Here's how the part is built. I have some questions about the finished solid (model axes, mm). A direction names the side the tool comes from. Coordinates: 2 decimals unless noted, no trailing zeros. Write each loop counter-clockwise with the first axis right and the second up, starting at its lowest first coordinate (ties: lowest second). Pieces come first, ordered by that corner, then holes.
Item 1: If we mould it in two halves opening along Y, with no side actions, what happens to faces 4 (the face through (8, 20, 4)), 5 (the face through (-6, 37, -122)), 6 (the face through (1.52, 64.59, -103.96))? For each: pulls with the +Y half, pulls with the -Y half, needs draft (parallel to the pull), parting line crosses it, or undercut.
Item 2: I want a section at C-C (x = 11.5). Please give me the cut outline in (y, z), and give its area (3 significant figures).
Item 3: I want a section at B-B (z = -86). Please give me the cut outline in (x, y).
Item 4: Please list where these lines run through material, in increasing order: line 1 (Y direction, x = 1.75, z = -94.5); line 2 (Z direction, x = 2.5, y = 69.5); line 3 (Y direction, x = 1.4, z = -27).
Item 5: For faces 1 (the face through (1.52, 22.15, -34.3)), 2 (the face through (8, 14, 0.975)), 3 (the face through (-3, 36.7, -125.4)), which set-ups out of +Z, -Z, +X, -X, +Y, -Y let a thin tool reach every point of the face, with its end or its side?
Item 6: I want a section at A-A (y = -10.68). Please give me the cut outline in (x, z).
Item 7: I'm going to push flat-ended pins straight in: P1, Ø6.5, axis at y = 0, z = -120, coming from the +X side; P2, Ø1.8, axis at x = 9.5, z = 4.5, coming from the -Y side; P3, Ø2.5, axis at x = -2, z = -123, coming from the +Y side. Where does each tip first touch, or does it pass through?
from build123d import *

# Parameters (mm, degrees)
SKETCH_1_R          = 2
EXTRUDE_1_DEPTH     = 3
EXTRUDE_2_DEPTH     = 10
CUT_EXTRUDE_3_DEPTH = 4
CHAMFER_1_SIZE      = 1
EXTRUDE_3_DEPTH     = 6
SKETCH_11_W         = 3
SKETCH_11_H         = 14
CUT_EXTRUDE_4_DEPTH = 162.773826789
SKETCH_12_R         = 1.45
CUT_EXTRUDE_5_DEPTH = 157.648043168


with BuildPart() as part:
    # Sketch 1 → Extrude 1 (new body)
    with BuildSketch(Plane(origin=(0, 0, 0), x_dir=(0, 0, -1), z_dir=(1, 0, 0))):
        Polygon((0, -15.68), (127.277441161, -15.68), (127.277441161, 89.32), (-6.974965275, 89.32), (-6.974965275, -15.68), align=None)
        with Locations((0, -10.68)):
            Circle(SKETCH_1_R, mode=Mode.SUBTRACT)
        with Locations((27, -10.68)):
            Circle(SKETCH_1_R, mode=Mode.SUBTRACT)
        with Locations((27, 0)):
            Circle(SKETCH_1_R, mode=Mode.SUBTRACT)
        Circle(SKETCH_1_R, mode=Mode.SUBTRACT)
        with Locations((93, 0)):
            Circle(SKETCH_1_R, mode=Mode.SUBTRACT)
        with Locations((93, -10.68)):
            Circle(SKETCH_1_R, mode=Mode.SUBTRACT)
        with Locations((120, -10.68)):
            Circle(SKETCH_1_R, mode=Mode.SUBTRACT)
        with Locations((120, 0)):
            Circle(SKETCH_1_R, mode=Mode.SUBTRACT)
        with Locations((73.5, 73)):
            Circle(SKETCH_1_R, mode=Mode.SUBTRACT)
        with Locations((73.5, 83.68)):
            Circle(SKETCH_1_R, mode=Mode.SUBTRACT)
        with Locations((46.5, 83.68)):
            Circle(SKETCH_1_R, mode=Mode.SUBTRACT)
        with Locations((46.5, 73)):
            Circle(SKETCH_1_R, mode=Mode.SUBTRACT)
    extrude(amount=EXTRUDE_1_DEPTH)

    # Sketch 2 → Extrude 2 (add)
    with BuildSketch(Plane(origin=(3, 0, 0), x_dir=(0, 0, -1), z_dir=(1, 0, 0))):
        Polygon((-6.974965275, 20), (-6.974965275, 9.003796157), (-4.947379944, 9.003796157), (-0.974965275, 9.003796157), (-0.974965275, 20), (-4.947379944, 20), align=None)
    extrude(amount=EXTRUDE_2_DEPTH)

    # Sketch 9 → Cut-Extrude 3 (cut)
    with BuildSketch(Plane(origin=(3, 0, 0), x_dir=(0, 0, -1), z_dir=(1, 0, 0))):
        with BuildLine():
            Line((14.793826902, 53.360356634), (27.387336033, 65.953865765))
            ThreePointArc((27.387336033, 65.953865765), (27.387336033, 70.795026635), (22.546175163, 70.795026635))
            Line((22.546175163, 70.795026635), (9.952666032, 58.201517504))
            ThreePointArc((9.952666032, 58.201517504), (9.952666032, 53.360356634), (14.793826902, 53.360356634))
        make_face()
        with BuildLine():
            Line((20.897912876, 31.977379799), (40.129928133, 51.209395056))
            ThreePointArc((40.129928133, 51.209395056), (40.129928133, 58.660989456), (32.678333733, 58.660989456))
            Line((32.678333733, 58.660989456), (13.446318476, 39.428974199))
            ThreePointArc((13.446318476, 39.428974199), (13.446318476, 31.977379799), (20.897912876, 31.977379799))
        make_face()
        with BuildLine():
            Line((20.319435032, 8.171706676), (48.67938199, 36.531653634))
            ThreePointArc((48.67938199, 36.531653634), (48.67938199, 41.992648329), (43.218387294, 41.992648329))
            Line((43.218387294, 41.992648329), (14.858440337, 13.632701372))
            ThreePointArc((14.858440337, 13.632701372), (14.858440337, 8.171706676), (20.319435032, 8.171706676))
        make_face()
        Polygon((-6.974965275, 69.32), (13.025034725, 89.32), (-6.974965275, 89.32), align=None)
        with BuildLine():
            ThreePointArc((60.151237943, 62.780937069), (56.651237943, 59.280937069), (60.151237943, 55.780937069))
            Line((60.151237943, 55.780937069), (60.151237943, 62.780937069))
        make_face()
        with BuildLine():
            Line((60.151237943, 62.780937069), (60.151237943, 55.780937069))
            ThreePointArc((60.151237943, 55.780937069), (62.626111677, 56.806063335), (63.651237943, 59.280937069))
            ThreePointArc((63.651237943, 59.280937069), (62.626111677, 61.755810803), (60.151237943, 62.780937069))
        make_face()
        with BuildLine():
            ThreePointArc((60.151237943, 40.32), (56.651237943, 36.82), (60.151237943, 33.32))
            Line((60.151237943, 33.32), (60.151237943, 40.32))
        make_face()
        with BuildLine():
            Line((60.151237943, 40.32), (60.151237943, 33.32))
            ThreePointArc((60.151237943, 33.32), (62.626111677, 34.345126266), (63.651237943, 36.82))
            ThreePointArc((63.651237943, 36.82), (62.626111677, 39.294873734), (60.151237943, 40.32))
        make_face()
        with BuildLine():
            ThreePointArc((60.151237943, 10.666059051), (56.651237943, 7.166059051), (60.151237943, 3.666059051))
            Line((60.151237943, 3.666059051), (60.151237943, 10.666059051))
        make_face()
        with BuildLine():
            Line((60.151237943, 10.666059051), (60.151237943, 3.666059051))
            ThreePointArc((60.151237943, 3.666059051), (62.626111677, 4.691185317), (63.651237943, 7.166059051))
            ThreePointArc((63.651237943, 7.166059051), (62.626111677, 9.640932785), (60.151237943, 10.666059051))
        make_face()
        with BuildLine():
            ThreePointArc((71.623093896, 36.531653634), (71.623093896, 41.992648329), (77.084088591, 41.992648329))
            Line((77.084088591, 41.992648329), (105.444035549, 13.632701372))
            ThreePointArc((105.444035549, 13.632701372), (105.444035549, 8.171706676), (99.983040853, 8.171706676))
            Line((99.983040853, 8.171706676), (71.623093896, 36.531653634))
        make_face()
        with BuildLine():
            ThreePointArc((80.172547753, 51.209395056), (80.172547753, 58.660989456), (87.624142153, 58.660989456))
            Line((87.624142153, 58.660989456), (106.85615741, 39.428974199))
            ThreePointArc((106.85615741, 39.428974199), (106.85615741, 31.977379799), (99.40456301, 31.977379799))
            Line((99.40456301, 31.977379799), (80.172547753, 51.209395056))
        make_face()
        with BuildLine():
            ThreePointArc((92.915139853, 65.953865765), (92.915139853, 70.795026635), (97.756300723, 70.795026635))
            Line((97.756300723, 70.795026635), (110.349809854, 58.201517504))
            ThreePointArc((110.349809854, 58.201517504), (110.349809854, 53.360356634), (105.508648984, 53.360356634))
            Line((105.508648984, 53.360356634), (92.915139853, 65.953865765))
        make_face()
        Polygon((127.277441161, 89.32), (107.277441161, 89.32), (127.277441161, 69.32), align=None)
    extrude(amount=-CUT_EXTRUDE_3_DEPTH, mode=Mode.SUBTRACT)

    # Chamfer 1
    chamfer_1_edges = [part.edges().sort_by_distance(p)[0] for p in [
        (3, 73, -44.5),
        (3, 83.68, -44.5),
        (3, 83.68, -71.5),
        (3, 73, -71.5),
        (3, 0, -118),
        (3, -10.68, -91),
        (3, 0, -91),
        (3, 0, 2),
        (3, 0, -25),
        (3, -10.68, -25),
        (3, -10.68, -118),
        (3, -10.68, 2),
    ]]
    chamfer(chamfer_1_edges, length=CHAMFER_1_SIZE)

    # Sketch 10 → Extrude 3 (add)
    with BuildSketch(Plane.ZY):
        Polygon((-127.277441161, 36.82), (-127.277441161, 46.82), (-120.277441161, 46.82), (-120.277441161, 26.82), (-127.277441161, 26.82), align=None)
        Polygon((-0.025034725, 26.82), (6.974965275, 26.82), (6.974965275, 36.82), (6.974965275, 46.82), (-0.025034725, 46.82), align=None)
    extrude(amount=EXTRUDE_3_DEPTH)

    # Sketch 11 → Cut-Extrude 4 (cut, through all)
    with BuildSketch(Plane(origin=(0, 0, -127.277441161), x_dir=(-1, 0, 0), z_dir=(0, 0, -1))):
        with Locations((1.5, 36.82)):
            Rectangle(SKETCH_11_W, SKETCH_11_H)
    extrude(amount=-CUT_EXTRUDE_4_DEPTH, mode=Mode.SUBTRACT)

    # Sketch 12 → Cut-Extrude 5 (cut, through all)
    with BuildSketch(Plane.ZY.offset(6)):
        with Locations((-123.777441161, 36.82)):
            Circle(SKETCH_12_R)
        with Locations((3.474965275, 36.82)):
            Circle(SKETCH_12_R)
    extrude(amount=-CUT_EXTRUDE_5_DEPTH, mode=Mode.SUBTRACT)


solid = part.part
Answer:
1. face 4: pulls with the +Y half
1. face 5: needs draft
1. face 6: undercut
2. outline: (9, 0.97) - (20, 0.97) - (20, 6.97) - (9, 6.97) - close
2. area: 66.0 mm2
3. outline: (0, -15.68) - (3, -15.68) - (3, 22.15) - (0, 22.15) - close; (0, 33.08) - (3, 33.08) - (3, 45.38) - (0, 45.38) - close; (0, 59.77) - (3, 59.77) - (3, 89.32) - (0, 89.32) - close
4. line 1: y = -15.68 to -12, -9.36 to -1.32, 1.32 to 13.65, 24.58 to 36.88, 51.79 to 64.37, 71.69 to 89.32
4. line 2: z = -127.1 to -99.05, -92.1 to -28.2, -21.25 to 6.79
4. line 3: y = -15.68 to -12.68, -8.68 to -2, 2 to 14.85, 25.77 to 38.08, 52.98 to 65.57, 71.13 to 89.32
5. face 1: +X, -X
5. face 2: -Z, +X, +Y, -Y
5. face 3: +Z, -Z
6. outline: (0, -127.28) - (3, -127.28) - (3, -123) - (2, -122) - (0, -122) - close; (0, -118) - (2, -118) - (3, -117) - (3, -96) - (2, -95) - (0, -95) - close; (0, -91) - (2, -91) - (3, -90) - (3, -30) - (2, -29) - (0, -29) - close; (0, -25) - (2, -25) - (3, -24) - (3, -3) - (2, -2) - (0, -2) - close; (0, 2) - (2, 2) - (3, 3) - (3, 6.97) - (0, 6.97) - close
7. P1: stops at x = 3
7. P2: stops at y = 9
7. P3: stops at y = 46.82
